Can you work these out from the drawing? Everything is in mm from the part's minimum corner. A direction names the side the tool comes from. Give positions to 0.01 mm unless a question says otherwise; leave off trailing zeros. Loops run counter-clockwise (first coordinate to the right, second up) from the corner with the lowest first, then second, coordinate; pieces in that order, holes last. Notation, with made-up numbers: (9.5, 36) -> (62.5, 36) arc R19 ccw to (62.5, 66) -> close; hole circle Ø5 at (61, 55). An arc over 180 degrees is marked (long way). Return JSON: item names as keys, results as strings. Group by question number.
Q1. Will these pins go through, and if not, where does the flat tip stop? pin 1 (1 mm diameter, centred on x = 13.5, z = 4, fed in from -Y); pin 2 (2 mm diameter, centred on x = 15.5, z = 2, fed in from +Y); pin 3 (2 mm diameter, centred on x = 11.5, z = 1.5, fed in from +Y); pin 4 (2.5 mm diameter, centred on x = 17.36, z = 2.96, fed in from +Y).
Q2. Suppose I cut it at D-D, the plane z = 5.5. Please give me the cut outline in (x, y) (1 decimal).
Q3. Thinking about a two-plate mould opening in Z: for the marked faces 4, 5 and 6, which applies, pulls with the +Z half, pulls with the -Z half, needs draft (parallel to the pull), parting line crosses it, or undercut?
Q4. Suppose I cut it at A-A, the plane y = 9. Please give me the cut outline in (x, z) (1 decimal).
Q5. Suppose I cut it at C-C, the plane z = 3.5. Please give me the cut outline in (x, y) (1 decimal).
Q6. I need wall thicknesses on line 1 along Y through (x, z) = (16.75, 4.85); line 2 along Y through (x, z) = (6, 0.5) (1 decimal); line 3 along X through (y, z) = (12, 5.1) (1 decimal). Which ranges of each line are inside material? Lowest first, please. Write a range as [from, to].
Q7. Suppose I cut it at B-B, the plane x = 2.25. Please give me the cut outline in (y, z), and give its area (3 significant figures).
Q8. Which directions (+Z, -Z, +X, -X, +Y, -Y) give clear straight access to the entire face, cutting with the end or side of a thin tool? Please do the marked faces 1, 2 and 3.
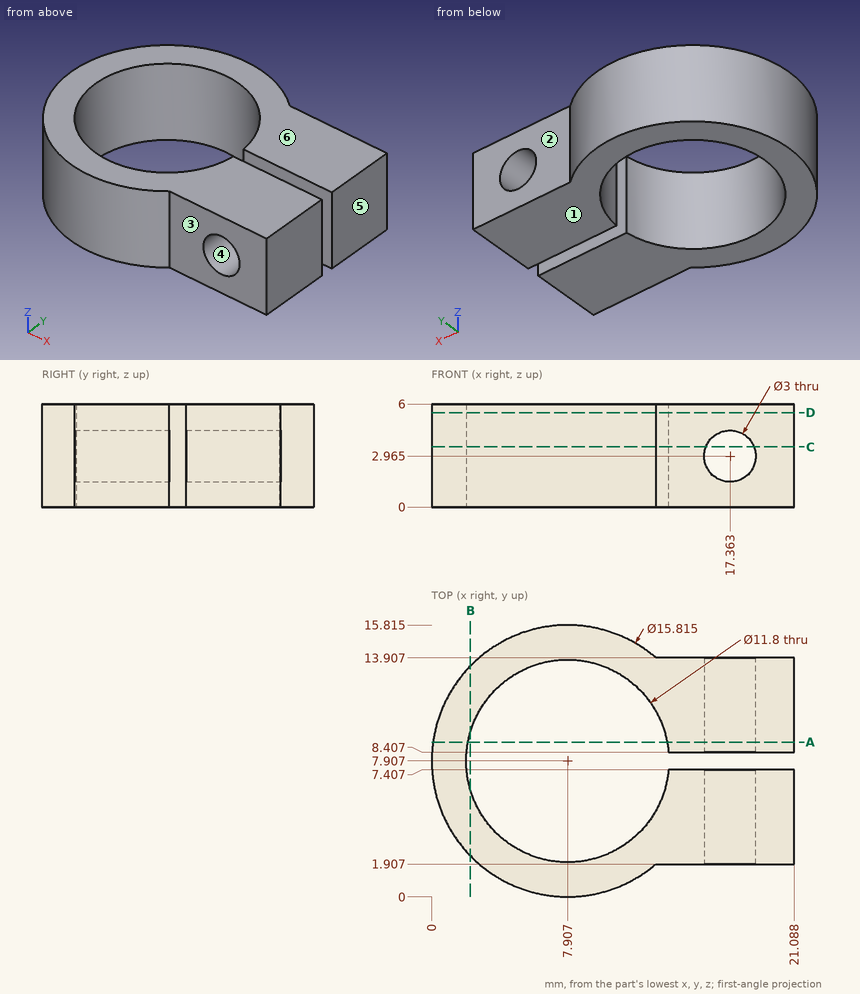
Ans:
{
 "1": {"pin 1": "stops at y = 1.86", "pin 2": "stops at y = 13.91", "pin 3": "stops at y = 15.38", "pin 4": "passes through"},
 "2": {"outline": "(13.1, 1.9) -> (21.1, 1.9) -> (21.1, 7.4) -> (13.8, 7.4) arc R5.9 cw (long way) to (13.8, 8.4) -> (21.1, 8.4) -> (21.1, 13.9) -> (13.1, 13.9) arc R7.9 ccw (long way) to start"},
 "3": {"face 4": "undercut", "face 5": "needs draft", "face 6": "pulls with the +Z half"},
 "4": {"outline": "(0.1, 0) -> (2.1, 0) -> (2.1, 6) -> (0.1, 6) -> close; (13.7, 0) -> (21.1, 0) -> (21.1, 6) -> (13.7, 6) -> close; hole circle Ø3 at (17.4, 3)"},
 "5": {"outline": "(13.1, 1.9) -> (16, 1.9) -> (16, 7.4) -> (13.8, 7.4) arc R5.9 cw (long way) to (13.8, 8.4) -> (16, 8.4) -> (16, 13.9) -> (13.1, 13.9) arc R7.9 ccw (long way) to start; (18.8, 1.9) -> (21.1, 1.9) -> (21.1, 7.4) -> (18.8, 7.4) -> close; (18.8, 8.4) -> (21.1, 8.4) -> (21.1, 13.9) -> (18.8, 13.9) -> close"},
 "6": {"line 1": "y = [1.91, 7.41], [8.41, 13.91]", "line 2": "y = [0.2, 2.3], [13.5, 15.6]", "line 3": "x = [1.1, 3.7], [12.2, 21.1]"},
 "7": {"outline": "(2.38, 0) -> (6.23, 0) -> (6.23, 6) -> (2.38, 6) -> close; (9.58, 0) -> (13.43, 0) -> (13.43, 6) -> (9.58, 6) -> close", "area": "46.2 mm^2"},
 "8": {"face 1": "-Z, +X, -X, +Y, -Y", "face 2": "+Z, -Z, +X, +Y", "face 3": "+Z, -Z, +X, -Y"}
}
